Design review of the part built by this model. Coordinates are the model's own, in mm. A direction names the side the tool comes from. Give positions to 0.01 mm unless a question says otherwise; leave off trailing zeros. Write each loop counter-clockwise with the first axis right and the second up, starting at its lowest first coordinate (ties: lowest second). Pieces come first, ordered by that corner, then holes. Notation, with made-up numbers: M 39,66.25 L 65,66.25 A6 ccw 65,77.25 Z; hole C 44,83.5 d10. An arc over 180 degrees is marked long. Answer in a Markdown table with one row per item.
```python
from build123d import *

# Parameters (mm, degrees)
SKETCH_1_W                   = 57
SKETCH_1_H                   = 18
HOLE_WIZARD_M100_1_D         = 104
HOLE_WIZARD_M100_1_DEPTH     = 1.5
SKETCH_4_W                   = 10
SKETCH_4_H                   = 15
HOLE_WIZARD_M8_1_D           = 10
HOLE_WIZARD_M8_1_CBORE_D     = 104
HOLE_WIZARD_M8_1_CBORE_DEPTH = 1.5
HOLE_WIZARD_5_2_5_2_1_REACH  = 93.449
HOLE_WIZARD_5_2_5_2_1_BORE_R = 2.6
HOLE_WIZARD_25_0_25_1_D      = 25
HOLE_WIZARD_25_0_25_1_DEPTH  = 30


with BuildPart() as part:
    # 草图1 → 旋转1 (revolve)
    with BuildSketch(Plane.XZ, mode=Mode.PRIVATE) as revolve_1_sk:
        with Locations((28.5, 0)):
            Rectangle(SKETCH_1_W, SKETCH_1_H)
    revolve(revolve_1_sk.sketch.rotate(Axis((0, 0, 9), (0, 0, -1)), 180), axis=Axis((0, 0, 9), (0, 0, -1)))

    # M100 间隙孔1
    with Locations(Plane.XY.offset(9)):
        with Locations((0, 0)):
            Hole(HOLE_WIZARD_M100_1_D / 2, depth=HOLE_WIZARD_M100_1_DEPTH)

    # 草图4 → 旋转2 (revolve)
    with BuildSketch(Plane.XZ):
        with Locations((5, 15)):
            Rectangle(SKETCH_4_W, SKETCH_4_H)
    revolve(axis=Axis((0, 0, 22.5), (0, 0, -1)))

    # M8 六角头螺栓的柱形沉头孔1 (through all)
    with Locations(Plane(origin=(0, 0, -9), x_dir=(-1, 0, 0), z_dir=(0, 0, -1))):
        with Locations((0, 0)):
            CounterBoreHole(HOLE_WIZARD_M8_1_D / 2, HOLE_WIZARD_M8_1_CBORE_D / 2, HOLE_WIZARD_M8_1_CBORE_DEPTH)

    # Ø5.2 (5.2) 直径孔1 bore (on position points) → Ø5.2 (5.2) 直径孔1 (cut, up to next)
    with BuildSketch(Plane(origin=(0, -10, 16), x_dir=(-1, 0, 0), z_dir=(0, -1, 0)), mode=Mode.PRIVATE) as hole_wizard_5_2_5_2_1_sk1:
        Circle(HOLE_WIZARD_5_2_5_2_1_BORE_R)
    hole_wizard_5_2_5_2_1_tool1 = extrude(hole_wizard_5_2_5_2_1_sk1.sketch, amount=-HOLE_WIZARD_5_2_5_2_1_REACH, mode=Mode.PRIVATE) & part.part
    add(hole_wizard_5_2_5_2_1_tool1.solids().sort_by_distance((0, -10, 16))[0], mode=Mode.SUBTRACT)

    # Ø25.0 (25) 直径孔1
    with Locations(Plane(origin=(0, 0, -7.5), x_dir=(-1, 0, 0), z_dir=(0, 0, -1))):
        with Locations((-30, 0), (-15, 25.980762114), (15, 25.980762114), (30, 0), (15, -25.980762114), (-15, -25.980762114)):
            Hole(HOLE_WIZARD_25_0_25_1_D / 2, depth=HOLE_WIZARD_25_0_25_1_DEPTH)


solid = part.part
```
1) Add section D-D (z = 11.5). Write out the cut boundary in (x, y), and give its area (3 significant figures).
Geometry says:
| item | result |
|---|---|
| outline | C 0,0 d20; hole C 0,0 d10 |
| area | 236 mm^2 |
2) To check wall thickness, follow probe 1 along Y at (x, z) = (-15, 2.5); probe 2 along Y at (x, z) = (0, 7.95); probe 3 along Y at (x, z) = (-6, -1.5). State the ranges of each line that lie inside material, in increasing order. Write a range as [from, to].
Geometry says:
| item | result |
|---|---|
| probe 1 | [-54.99, -38.48], [-13.48, 13.48], [38.48, 54.99] |
| probe 2 | [-57, -52], [-10, -5], [5, 10], [52, 57] |
| probe 3 | [-56.68, -34.66], [-17.31, 17.31], [34.66, 56.68] |
3) Add section B-B (z = -3). Write out the cut boundary in (x, y).
Geometry says:
| item | result |
|---|---|
| outline | C 0,0 d114; hole C -30,0 d25; hole C -15,-25.98 d25; hole C -15,25.98 d25; hole C 0,0 d10; hole C 15,-25.98 d25; hole C 15,25.98 d25; hole C 30,0 d25 |
4) For faces 5 (the face through (-11, 1, 7.5)), 6 (the face through (-11, 1, -7.5)), 7 (the face through (2.6, -7.2, 15.9)), list the 3-axis set-ups (+Z, -Z, +X, -X, +Y, -Y) from which the entire face can be reached by the end or side of a thin tool; tool diameter is ignored.
Geometry says:
| item | result |
|---|---|
| face 5 | +Z |
| face 6 | -Z |
| face 7 | -Y |
5) Add section C-C (x = 34.5). Write out the cut boundary in (y, z).
Geometry says:
| item | result |
|---|---|
| outline | M -45.37,-9 L -38.91,-9 L -38.91,-7.5 L -11.66,-7.5 L -11.66,7.5 L -38.91,7.5 L -38.91,9 L -45.37,9 Z; M 11.66,-7.5 L 38.91,-7.5 L 38.91,-9 L 45.37,-9 L 45.37,9 L 38.91,9 L 38.91,7.5 L 11.66,7.5 Z |
6) Add section A-A (x = -19). Write out the cut boundary in (y, z).
Geometry says:
| item | result |
|---|---|
| outline | M -53.74,-9 L -48.4,-9 L -48.4,-7.5 L -37.82,-7.5 L -37.82,7.5 L -48.4,7.5 L -48.4,9 L -53.74,9 Z; M -14.14,-7.5 L -5.94,-7.5 L -5.94,7.5 L -14.14,7.5 Z; M 5.94,-7.5 L 14.14,-7.5 L 14.14,7.5 L 5.94,7.5 Z; M 37.82,-7.5 L 48.4,-7.5 L 48.4,-9 L 53.74,-9 L 53.74,9 L 48.4,9 L 48.4,7.5 L 37.82,7.5 Z |
7) Insertion check: P1, Ø7, axis at x = 0, z = 16, coming from the +Y side; P2, Ø4, axis at x = 40, y = -6, coming from the +Z side; P3, Ø2, axis at x = 34, y = 27, coming from the -Z side. Each pin has a flat end and moves straight along its axis. Give the tip position at first contact, or say it passes through.
Geometry says:
| item | result |
|---|---|
| P1 | y = 10 |
| P2 | z = 7.5 |
| P3 | z = -7.5 |
8) The part is to be moulded in two halves that separate along X. For faces 1 (the face through (-24.21, 34.43, 0.11)), 2 (the face through (46, -25, 9)), 3 (the face through (12.356, -55.645, 0.126)), 4 (the face through (-0.651, 4.957, 7.71)), say which applies: released by +X, released by -X, zero draft, split by the parting line, or undercut.
Geometry says:
| item | result |
|---|---|
| face 1 | undercut |
| face 2 | zero draft |
| face 3 | split by the parting line |
| face 4 | undercut |
